For this review, take the finished solid that the model builds, in its own axes (mm). A direction names the side the tool comes from. Give positions to 0.01 mm unless a question says otherwise; leave off trailing zeros. Write each loop counter-clockwise with the first axis right and the second up, starting at its lowest first coordinate (ties: lowest second). Pieces come first, ordered by that corner, then holes.
1) We need section A-A on x = 0. Give the boundary of the cut face in (y, z).
2) Machinability: for faces 4 (the face through (22, 3, 15)), 5 (the face through (-5, 3, -22)), 6 (the face through (-23, 3, 15)), 7 (the face through (22, 3, 5)), which of the approach directions +Z, -Z, +X, -X, +Y, -Y give a long, thin tool a straight path to every point of the face, cutting with its end or side? Answer none if there is none.
3) We need section C-C on x = 7.75. Give the boundary of the cut face in (y, z).
4) Wall thickness on line 1 along Z through (x, y) = (-7.75, 3.85); line 2 along X through (y, z) = (3, 0); line 3 along X through (y, z) = (2.6, -21): over which ranges is each line inside the solid? List them lowest first.
5) For P1, Ø2.5, axis at y = 1.5, z = 19.5, coming from the -X side; P2, Ø2.5, axis at x = 22.5, y = 2.5, coming from the +Z side; P3, Ø1.5, axis at x = -11.5, y = 2, coming from the -Z side, all flat-tipped, find the tip position at first contact; note any pin that passes through.
6) We need section B-B on z = -7. Give the boundary of the cut face in (x, y), and give its area (3 significant figures).
7) Draft analysis for pull direction Z (two halves, no side actions). For faces 1 (the face through (25, 2, 10)), 2 (the face through (10, 3, -20)), 3 (the face through (-8.119, 2.465, -11.764)), state which applies: pulls with the +Z half, pulls with the -Z half, needs draft (parallel to the pull), parting line crosses it, or undercut.
8) We need section D-D on y = 3.6. Give the number of separate pieces and of enclosed holes in the cut face, and give its area (3 significant figures).
from build123d import *

# Parameters (mm, degrees)
SKETCH_1_W          = 50
SKETCH_1_H          = 50
SKETCH_1_R          = 1.7
SKETCH_1_R_2        = 6.5
EXTRUDE_1_DEPTH     = 5
SKETCH_6_W          = 10
SKETCH_6_H          = 5
SKETCH_6_W_2        = 5
SKETCH_6_H_2        = 10
CUT_EXTRUDE_1_DEPTH = 6


with BuildPart() as part:
    # 草图1 → 凸台-拉伸1 (new body)
    with BuildSketch(Plane(origin=(0, 0, 0), x_dir=(1, 0, 0), z_dir=(0, 1, 0))):
        Rectangle(SKETCH_1_W, SKETCH_1_H)
        with Locations((-15.5, 0)):
            Circle(SKETCH_1_R, mode=Mode.SUBTRACT)
        with Locations((-7.75, 13.423393759)):
            Circle(SKETCH_1_R, mode=Mode.SUBTRACT)
        with Locations((7.75, 13.423393759)):
            Circle(SKETCH_1_R, mode=Mode.SUBTRACT)
        with Locations((15.5, 0)):
            Circle(SKETCH_1_R, mode=Mode.SUBTRACT)
        with Locations((7.75, -13.423393759)):
            Circle(SKETCH_1_R, mode=Mode.SUBTRACT)
        with Locations((-7.75, -13.423393759)):
            Circle(SKETCH_1_R, mode=Mode.SUBTRACT)
        with Locations((0, 7)):
            Circle(SKETCH_1_R_2, mode=Mode.SUBTRACT)
    extrude(amount=EXTRUDE_1_DEPTH)

    # 草图6 → 切除-拉伸1 (cut, through all)
    with BuildSketch(Plane(origin=(0, 5, 0), x_dir=(1, 0, 0), z_dir=(0, 1, 0))):
        with Locations((-10, 22.5)):
            Rectangle(SKETCH_6_W, SKETCH_6_H)
        with Locations((10, 22.5)):
            Rectangle(SKETCH_6_W, SKETCH_6_H)
        with Locations((-22.5, -20)):
            Rectangle(SKETCH_6_W_2, SKETCH_6_H_2)
        with Locations((-22.5, 0)):
            Rectangle(SKETCH_6_W_2, SKETCH_6_H_2)
        with Locations((22.5, -20)):
            Rectangle(SKETCH_6_W_2, SKETCH_6_H_2)
        with Locations((22.5, 0)):
            Rectangle(SKETCH_6_W_2, SKETCH_6_H_2)
    extrude(amount=-CUT_EXTRUDE_1_DEPTH, mode=Mode.SUBTRACT)


solid = part.part
Results list:
1. outline: (0, -25) - (5, -25) - (5, -13.5) - (0, -13.5) - close; (0, -0.5) - (5, -0.5) - (5, 25) - (0, 25) - close
2. face 4: +Z, +X, +Y, -Y
2. face 5: -Z, +Y, -Y
2. face 6: +Z, -X, +Y, -Y
2. face 7: +X, +Y, -Y
3. outline: (0, -20) - (5, -20) - (5, -15.12) - (0, -15.12) - close; (0, -11.72) - (5, -11.72) - (5, 11.72) - (0, 11.72) - close; (0, 15.12) - (5, 15.12) - (5, 25) - (0, 25) - close
4. line 1: z = -20 to -15.12, -11.72 to 11.72, 15.12 to 25
4. line 2: x = -20 to -17.2, -13.8 to 13.8, 17.2 to 20
4. line 3: x = -25 to -15, -5 to 5, 15 to 25
5. P1: stops at x = -20
5. P2: stops at z = 15
5. P3: stops at z = -20
6. outline: (-25, 0) - (-6.5, 0) - (-6.5, 5) - (-25, 5) - close; (6.5, 0) - (25, 0) - (25, 5) - (6.5, 5) - close
6. area: 185 mm2
7. face 1: needs draft
7. face 2: pulls with the -Z half
7. face 3: undercut
8. separate pieces: 1
8. enclosed holes: 7
8. area: 2,010 mm2
